Here's how the part is built. I have some questions about the finished solid (model axes, mm). Give positions to 0.01 mm unless a question says otherwise; leave off trailing zeros. Write each loop counter-clockwise with the first axis right and the second up, starting at its lowest first coordinate (ties: lowest second). Pieces come first, ordered by that corner, then holes. Notation, with made-up numbers: (59.5, 65.25) -> (104.5, 65.25) arc R15 ccw to (104.5, 80.25) -> close; hole circle Ø1 at (65.5, -29). An arc over 180 degrees is marked (long way). Use one line per item in the form item = value.
Autodesk Inventor part; units mm, degrees
ref_plane "nut_XY" through (0, 0, -1.1938) normal (0, 0, 1) x (1, 0, 0)
ref_plane "nut_YZ" through (0, 0, -1.1938) normal (1, 0, 0) x (0, 1, 0)
ref_plane "nut_ZX" through (0, 0, -1.1938) normal (0, 1, 0) x (0, 0, 1)
sketch "Sketch_1" plane through (0, 0, 0) normal (1, 0, 0) x (0, 1, 0)
  line L0 (0, -1.1938) -> (0, 1.1938)
  line L1 (0, 1.1938) -> (6.9977, 1.1938)
  line L2 (6.9977, 1.1938) -> (8.3972, 0.6844)
  line L3 (8.3972, 0.6844) -> (8.3972, -1.1938)
  line L4 (8.3972, -1.1938) -> (0, -1.1938)
  line L5 (0, -1.1938) -> (0, 1.1938)
revolve "Revolution1" add sketch "Sketch_1" angle 360 about axis through (0, 0, -1.1938) along (0, 0, -1)
sketch "Sketch_2" plane through (0, 0, 0) normal (0, 0, 1) x (1, 0, 0)
  line L0 (-13.9954, 13.9954) -> (-13.9954, -13.9954)
  line L1 (-13.9954, -13.9954) -> (13.9954, -13.9954)
  line L2 (13.9954, -13.9954) -> (13.9954, 13.9954)
  line L3 (13.9954, 13.9954) -> (-13.9954, 13.9954)
  line L4 (-8.001, 0) -> (-4.0401, -6.9977)
  line L5 (-4.0401, -6.9977) -> (4.0401, -6.9977)
  line L6 (4.0401, -6.9977) -> (8.001, 0)
  line L7 (8.001, 0) -> (4.0401, 6.9977)
  line L8 (4.0401, 6.9977) -> (-4.0401, 6.9977)
  line L9 (-4.0401, 6.9977) -> (-8.001, 0)
extrude "Extrusion1" cut sketch "Sketch_2" along normal mid plane 4.7752
sketch "Sketch3" plane through (4.0401, 6.9977, -1.1938) normal (0, 0, -1) x (-1, 0, 0)
  point P0 (4.0401, -6.9977)
hole "Drilling 1" at (0, 0, -1.1938) direction (0, 0, 1) diameter 10.106 depth 2.3876 countersink diameter 11.9888 countersink angle 90
ref_plane "nut_XY" through (0, 0, -1.1938) normal (0, 0, 1) x (1, 0, 0)
ref_plane "nut_YZ" through (0, 0, -1.1938) normal (1, 0, 0) x (0, 1, 0)
ref_plane "nut_ZX" through (0, 0, -1.1938) normal (0, 1, 0) x (0, 0, 1)
properties part number "AT503M"
Q1. Will these pins go through, and if not, where does the flat tip stop? pin 1 Ø1 at (x, y) = (-4, -2.5) entering from +Z; pin 2 Ø1 at (x, z) = (5, 0.5) entering from +Y.
Result set:
pin_1 = 1.19
pin_2 = 6.19
Q2. If we mould it in two halves opening along X, with no side actions, what happens to faces 1 (the face through (0, -6.998, 0)), 2 (the face through (3.075, -4.01, 0.481)), 3 (the face through (5.99, -3.55, -0.02))? For each: +X half, -X half, draft (parallel to the pull), parting line (faces both ways), or undercut.
Result set:
face_1 = draft
face_2 = undercut
face_3 = +X half
Q3. I want a section at A-A, the plane z = 0.3. Write out the boundary of the cut face in (x, y).
Result set:
outline = (-8, 0) -> (-4.04, -7) -> (4.04, -7) -> (8, 0) -> (4.04, 7) -> (-4.04, 7) -> close; hole circle Ø10.11 at (0, 0)
Q4. I want a section at B-B, the plane z = -0.9. Write out the boundary of the cut face in (x, y), and give its area (3 significant figures).
Result set:
outline = (-8, 0) -> (-4.04, -7) -> (4.04, -7) -> (8, 0) -> (4.04, 7) -> (-4.04, 7) -> close; hole circle Ø11.4 at (0, 0)
area = 66.4 mm2
Q5. If I drill on line 1 along Y through (x, z) = (0, 0.5); line 2 along X through (y, z) = (3.75, 0.4); line 3 along X through (y, z) = (-1.25, -0.2), over which ranges is the centre line in solid material (lowest first)? Write a range as from..to.
Result set:
line_1 = -7..-5.05, 5.05..7
line_2 = -5.88..-3.39, 3.39..5.88
line_3 = -7.29..-4.9, 4.9..7.29
